```python
from build123d import *

# Parameters (mm, degrees)
BOSS_EXTRUDE1_DEPTH = 4
SKETCH2_R           = 1.5
BOSS_EXTRUDE2_DEPTH = 9


with BuildPart() as part:
    # Sketch1 → Boss-Extrude1 (new body)
    with BuildSketch(Plane(origin=(0, 0, 0), x_dir=(1, 0, 0), z_dir=(0, 1, 0))):
        Polygon((3.175426481, 0), (1.58771324, 2.75), (-1.58771324, 2.75), (-3.175426481, 0), (-1.58771324, -2.75), (1.58771324, -2.75), align=None)
    extrude(amount=BOSS_EXTRUDE1_DEPTH)

    # Sketch2 → Boss-Extrude2 (add)
    with BuildSketch(Plane.XZ):
        with Locations(Location((0, 0, 0), (0, 0, 270))):
            Circle(SKETCH2_R)
    extrude(amount=BOSS_EXTRUDE2_DEPTH)


solid = part.part
```
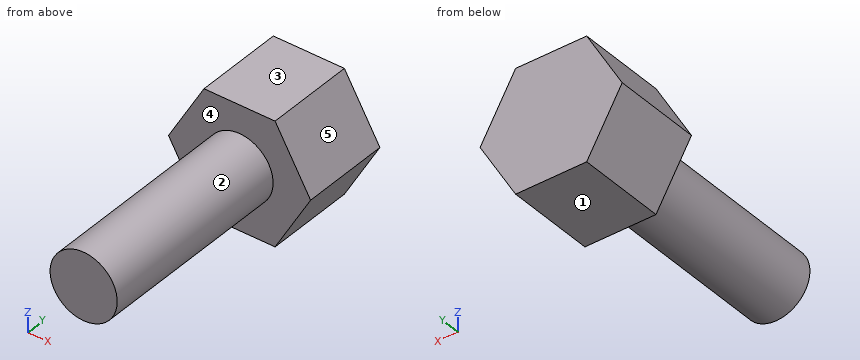
Input: part model. Units: mm. Frame: model coordinates. Face numbers are marked on the shaded views. A direction names the side the tool comes from. Give positions to 0.01 mm unless a question says otherwise; leave off trailing zeros. Order: outer loops, then holes, each group sorted by start corner. A loop starts at its lowest first (then second) coordinate and runs counter-clockwise, first axis right, second up.
1. Material intervals for L1, parallel to Y at x = 2, z = -1.5; L2, parallel to X at y = 0.5, z = 1.6; L3, parallel to Z at x = 1.25, y = -6, sorted ascending.
Derived:
L1: y = 0 to 4
L2: x = -2.25 to 2.25
L3: z = -0.83 to 0.83
2. Reachability of the marked faces 4 and 5 from +Z, -Z, +X, -X, +Y, -Y: full face, straight path, thin tool, end or side. Return the list, or none.
Derived:
face 4: -Y
face 5: +Z, +X, +Y, -Y
3. Section C-C on z = 0.9. Return the cut outline in (x, y), and give its area (3 significant figures).
Derived:
outline: (-2.66, 0) - (-1.2, 0) - (-1.2, -9) - (1.2, -9) - (1.2, 0) - (2.66, 0) - (2.66, 4) - (-2.66, 4) - close
area: 42.8 mm2
4. Pin query (flat end, axial travel): pin 1 (3 mm diameter, centred on y = -2, z = 1.5, fed in from +X); pin 2 (2 mm diameter, centred on x = -2, y = 2, fed in from -Z). Return the tip coordinate at first contact, or that it passes through.
Derived:
pin 1: stops at x = 1.5
pin 2: stops at z = -2.75
5. Section D-D on y = -0.75. Return the cut outline in (x, z), and give its area (3 significant figures).
Derived:
outline: circle Ø3 at (0, 0)
area: 7.07 mm2
6. Mould query, pull axis Z, two halves, no side actions, for the marked faces 1, 2 and 3. Classes: released by +Z, released by -Z, zero draft, split by the parting line, or undercut.
Derived:
face 1: released by -Z
face 2: split by the parting line
face 3: released by +Z
7. Section B-B on y = 2.25. Return the cut outline in (x, z), and give its area (3 significant figures).
Derived:
outline: (-3.18, 0) - (-1.59, -2.75) - (1.59, -2.75) - (3.18, 0) - (1.59, 2.75) - (-1.59, 2.75) - close
area: 26.2 mm2
8. Section A-A on x = 0. Return the cut outline in (y, z), and give its area (3 significant figures).
Derived:
outline: (-9, -1.5) - (0, -1.5) - (0, -2.75) - (4, -2.75) - (4, 2.75) - (0, 2.75) - (0, 1.5) - (-9, 1.5) - close
area: 49.0 mm2
